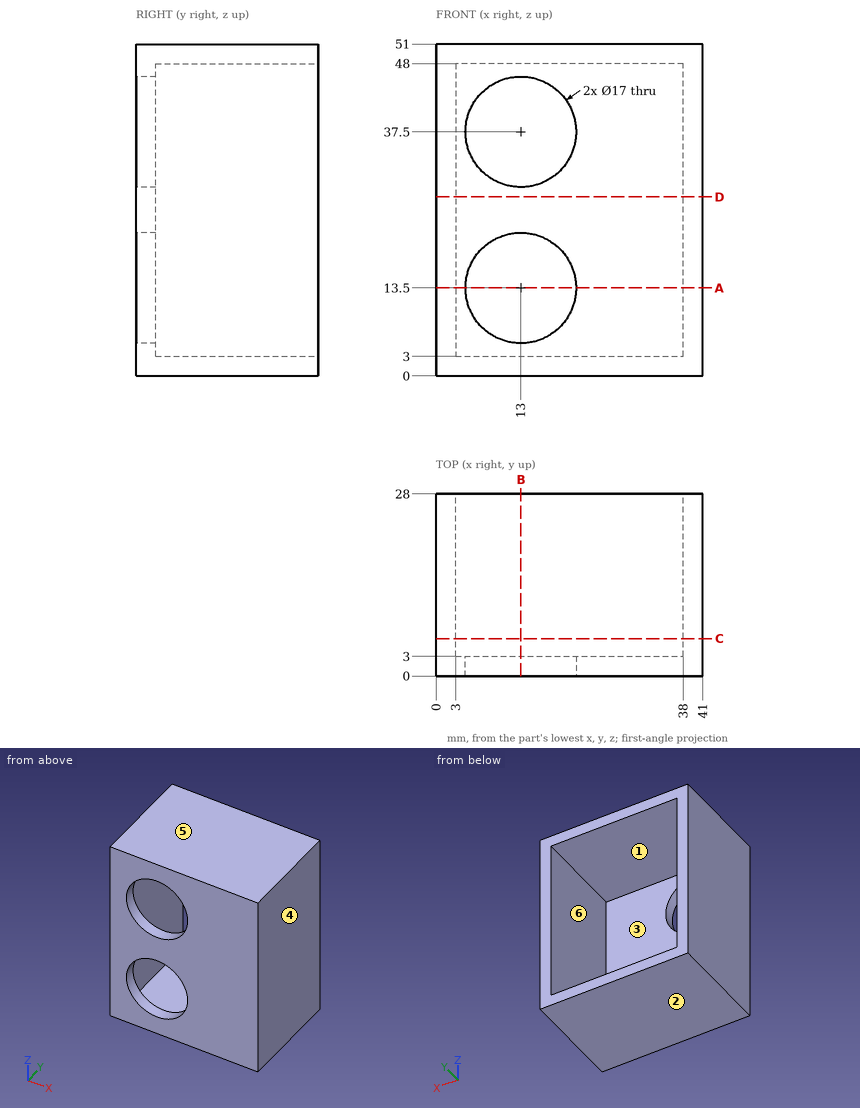
Job drawing, mm, ordinate dimensions from the low corner. One solid piece. A direction names the side the tool comes from. Round coordinates to 2 decimals unless told otherwise and drop trailing zeros. Write each loop counter-clockwise with the first axis right and the second up, starting at its lowest first coordinate (ties: lowest second). Pieces come first, ordered by that corner, then holes.
1) Band-saw the part on C-C, the plane y = 5.75. List the corners of the cut face in (x, z).
2) Band-saw the part on B-B, the plane x = 13. List the corners of the cut face in (y, z), and give its area (3 significant figures).
3) Band-saw the part on A-A, the plane z = 13.5. List the corners of the cut face in (x, y), and give its area (3 significant figures).
4) Mould opens along Z. For the marked faces 3, 4, 5 and 6 say: +Z half, -Z half, draft (parallel to the pull), parting line (faces both ways), or undercut.
5) 3-axis set-ups, long thin cutter, end or side, ignore diameter. For the marked faces 1 and 2: which of +Z, -Z, +X, -X, +Y, -Y reach the whole face in a straight line?
6) Drill centre lines: probe 1 along Z at (x, y) = (13, 1.55); probe 2 along X at (y, z) = (23.25, 35.5); probe 3 along Z at (x, y) = (5.5, 14.25). Where is each one in solid material? Low to high.
7) Band-saw the part on D-D, the plane z = 27.5. List the corners of the cut face in (x, y).
8) Pin check, flat tip, straight feed: pin 1 (13.5 mm diameter, centred on x = 13, z = 37.5, fed in from +Y). Stop position of the tip, or through.
Ans:
1. outline: (0, 0) - (41, 0) - (41, 51) - (0, 51) - close; hole (3, 3) - (38, 3) - (38, 48) - (3, 48) - close
2. outline: (0, 0) - (28, 0) - (28, 3) - (3, 3) - (3, 5) - (0, 5) - close; (0, 22) - (3, 22) - (3, 29) - (0, 29) - close; (0, 46) - (3, 46) - (3, 48) - (28, 48) - (28, 51) - (0, 51) - close
2. area: 201 mm2
3. outline: (0, 0) - (4.5, 0) - (4.5, 3) - (3, 3) - (3, 28) - (0, 28) - close; (21.5, 0) - (41, 0) - (41, 28) - (38, 28) - (38, 3) - (21.5, 3) - close
3. area: 222 mm2
4. face 3: undercut
4. face 4: draft
4. face 5: +Z half
4. face 6: undercut
5. face 1: +Y
5. face 2: -Z, +X, -X, +Y, -Y
6. probe 1: z = 0 to 5, 22 to 29, 46 to 51
6. probe 2: x = 0 to 3, 38 to 41
6. probe 3: z = 0 to 3, 48 to 51
7. outline: (0, 0) - (41, 0) - (41, 28) - (38, 28) - (38, 3) - (3, 3) - (3, 28) - (0, 28) - close
8. pin 1: passes through
